Verification items for the finished model (mm, model axes). Round coordinates to 2 decimals unless told otherwise and drop trailing zeros. Write each loop counter-clockwise with the first axis right and the second up, starting at its lowest first coordinate (ties: lowest second). Pieces come first, ordered by that corner, then holes. Notation, with made-up numbers: (67.5, -0.5) - (100.5, -0.5) arc R15 ccw to (100.5, 9.5) - close; hole circle Ø3 at (17, -12). An arc over 180 degrees is marked (long way). Answer as a JSON object with one key per item and string values.
```python
from build123d import *

# Parameters (mm, degrees)
CROQUIS1_R              = 1.5
CROQUIS1_RX             = 8
CROQUIS1_RY             = 5
CROQUIS1_W              = 10
CROQUIS1_H              = 14
CROQUIS1_W_2            = 12
CROQUIS1_H_2            = 7.5
SALIENTE_EXTRUIR1_DEPTH = 3


with BuildPart() as part:
    # Croquis1 → Saliente-Extruir1 (new body)
    with BuildSketch(Plane(origin=(0, 0, 0), x_dir=(1, 0, 0), z_dir=(0, 1, 0))):
        with BuildLine():
            Line((40.75, -26.5), (40.75, 23))
            ThreePointArc((40.75, 23), (39.724873734, 25.474873734), (37.25, 26.5))
            Line((37.25, 26.5), (-37.25, 26.5))
            ThreePointArc((-37.25, 26.5), (-39.724873734, 25.474873734), (-40.75, 23))
            Line((-40.75, 23), (-40.75, -26.5))
            Line((-40.75, -26.5), (-39.75, -33.5))
            Line((-39.75, -33.5), (39.75, -33.5))
            Line((39.75, -33.5), (40.75, -26.5))
        make_face()
        with Locations((34.25, 17)):
            Circle(CROQUIS1_R, mode=Mode.SUBTRACT)
        with Locations((-34.25, 17)):
            Circle(CROQUIS1_R, mode=Mode.SUBTRACT)
        with Locations((34.45, -13.75)):
            Circle(CROQUIS1_R, mode=Mode.SUBTRACT)
        with Locations((25.75, -16)):
            Circle(CROQUIS1_R, mode=Mode.SUBTRACT)
        with Locations((23.25, -26.5)):
            Circle(CROQUIS1_R, mode=Mode.SUBTRACT)
        with Locations((25.75, 8.5)):
            Circle(CROQUIS1_R, mode=Mode.SUBTRACT)
        with Locations((21.75, 19)):
            Circle(CROQUIS1_R, mode=Mode.SUBTRACT)
        with Locations((11.25, -3.5)):
            Circle(CROQUIS1_R, mode=Mode.SUBTRACT)
        with Locations((-28.75, -3.5)):
            Circle(CROQUIS1_R, mode=Mode.SUBTRACT)
        with Locations((0.75, -26.5)):
            Circle(CROQUIS1_R, mode=Mode.SUBTRACT)
        with Locations((0.75, 19.5)):
            Circle(CROQUIS1_R, mode=Mode.SUBTRACT)
        with Locations((-34.25, -14.5)):
            Circle(CROQUIS1_R, mode=Mode.SUBTRACT)
        with Locations((-8.75, -3.5)):
            Ellipse(CROQUIS1_RX, CROQUIS1_RY, mode=Mode.SUBTRACT)
        with Locations((34.75, 7.75)):
            Rectangle(CROQUIS1_W, CROQUIS1_H, mode=Mode.SUBTRACT)
        with BuildLine():
            Line((-1.658013335, 4.744885232), (12.795993333, 16.65752809))
            ThreePointArc((12.795993333, 16.65752809), (14.90752809, 16.454006667), (14.704006667, 14.34247191))
            Line((14.704006667, 14.34247191), (0.25, 2.429829053))
            ThreePointArc((0.25, 2.429829053), (-1.861534757, 2.633350475), (-1.658013335, 4.744885232))
        make_face(mode=Mode.SUBTRACT)
        with BuildLine():
            Line((-1.658013335, -11.744885232), (12.795993333, -23.65752809))
            ThreePointArc((12.795993333, -23.65752809), (14.90752809, -23.454006667), (14.704006667, -21.34247191))
            Line((14.704006667, -21.34247191), (0.25, -9.429829053))
            ThreePointArc((0.25, -9.429829053), (-1.861534757, -9.633350475), (-1.658013335, -11.744885232))
        make_face(mode=Mode.SUBTRACT)
        with BuildLine():
            Line((-15.841986665, -11.744885232), (-30.295993333, -23.65752809))
            ThreePointArc((-30.295993333, -23.65752809), (-32.40752809, -23.454006667), (-32.204006667, -21.34247191))
            Line((-32.204006667, -21.34247191), (-17.75, -9.429829053))
            ThreePointArc((-17.75, -9.429829053), (-15.638465243, -9.633350475), (-15.841986665, -11.744885232))
        make_face(mode=Mode.SUBTRACT)
        with BuildLine():
            Line((-15.841986665, 4.744885232), (-30.295993333, 16.65752809))
            ThreePointArc((-30.295993333, 16.65752809), (-32.40752809, 16.454006667), (-32.204006667, 14.34247191))
            Line((-32.204006667, 14.34247191), (-17.75, 2.429829053))
            ThreePointArc((-17.75, 2.429829053), (-15.638465243, 2.633350475), (-15.841986665, 4.744885232))
        make_face(mode=Mode.SUBTRACT)
        with BuildLine():
            Line((-19.142857143, -27.5), (-16.142857143, -27.5))
            ThreePointArc((-16.142857143, -27.5), (-14.642857143, -29), (-16.142857143, -30.5))
            Line((-16.142857143, -30.5), (-19.142857143, -30.5))
            ThreePointArc((-19.142857143, -30.5), (-20.642857143, -29), (-19.142857143, -27.5))
        make_face(mode=Mode.SUBTRACT)
        with Locations((-17.5, 16.25)):
            Rectangle(CROQUIS1_W_2, CROQUIS1_H_2, mode=Mode.SUBTRACT)
    extrude(amount=SALIENTE_EXTRUIR1_DEPTH)


solid = part.part
```
1. Cross-section at A-A (x = -34.25). Record the boundary of the cut face in (y, z).
Completed:
{"outline": "(0, -26.5) - (3, -26.5) - (3, -18.5) - (0, -18.5) - close; (0, -15.5) - (3, -15.5) - (3, 13) - (0, 13) - close; (0, 16) - (3, 16) - (3, 33.5) - (0, 33.5) - close"}
2. Material ranges on probe 1 along X at (y, z) = (2, 3.5); probe 2 along Z at (x, y) = (37, 1.25); probe 3 along X at (y, z) = (0.6, -9), recorded low to high. Write a range as from..to.
Completed:
{"probe 1": "x = -40.75..-30.25, -27.25..-16.75, -0.75..9.75, 12.75..40.75", "probe 2": "z = -26.5..-14.75, -0.75..33.5", "probe 3": "x = -40.75..-25.72, -21..3.5, 8.22..24.34, 27.16..29.75, 39.75..40.75"}
3. Cross-section at C-C (z = 3.5). Count the separate pieces of the cut face and the enclosed holes in it, plus the area to 4 significant figures.
Completed:
{"separate pieces": "4", "enclosed holes": "0", "area": "178.5 mm^2"}
4. Cross-section at B-B (x = 34.45). Record the boundary of the cut face in (y, z).
Completed:
{"outline": "(0, -26.5) - (3, -26.5) - (3, -18.49) - (0, -18.49) - close; (0, -15.51) - (3, -15.51) - (3, -14.75) - (0, -14.75) - close; (0, -0.75) - (3, -0.75) - (3, 12.25) - (0, 12.25) - close; (0, 15.25) - (3, 15.25) - (3, 33.5) - (0, 33.5) - close"}
5. Mould release check, pull along X, two halves, no side actions. Record for faces 1 (the face through (-11.5, 1, -16)), 2 (the face through (40.75, 1, 2)), 3 (the face through (1, 1, -26.5)), 4 (the face through (-30.25, 1.48, 3.43)): released by +X, released by -X, zero draft, split by the parting line, or undercut.
Completed:
{"face 1": "undercut", "face 2": "released by +X", "face 3": "zero draft", "face 4": "undercut"}
6. Go/stop test with a flat-tipped pin: pin 1 (1.8 mm diameter, centred on x = 21.75, z = -19, fed in from +Y). Record where the tip stops, or that it passes through.
Completed:
{"pin 1": "passes through"}
